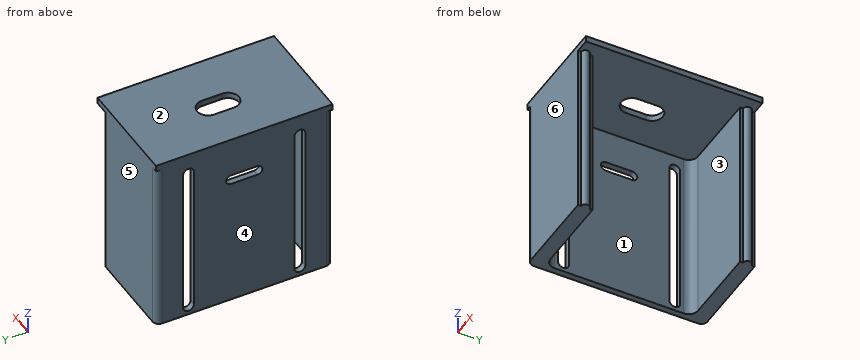
from build123d import *

# Parameters (mm, degrees)
CROQUIS1_W              = 34.637221952
CROQUIS1_H              = 57.24088581
SALIENTE_EXTRUIR1_DEPTH = 2
SALIENTE_EXTRUIR2_DEPTH = 57
CORTAR_EXTRUIR1_DEPTH   = 3
CORTAR_EXTRUIR2_DEPTH   = 6
CORTAR_EXTRUIR3_REACH   = 61


with BuildPart() as part:
    # Croquis1 → Saliente-Extruir1 (new body)
    with BuildSketch(Plane.XY):
        with Locations((-18.894886619, 25.199603339)):
            Rectangle(CROQUIS1_W, CROQUIS1_H)
    extrude(amount=SALIENTE_EXTRUIR1_DEPTH)

    # Croquis3 → Saliente-Extruir2 (add)
    with BuildSketch(Plane(origin=(0, 0, 0), x_dir=(-1, 0, 0), z_dir=(0, 0, -1))):
        with BuildLine():
            Line((6.325110646, 52.869153193), (6.325110646, 53.820046244))
            Line((6.325110646, 53.820046244), (34.213497595, 53.820046244))
            ThreePointArc((34.213497595, 53.820046244), (35.627711158, 53.234259806), (36.213497595, 51.820046244))
            Line((36.213497595, 51.820046244), (36.213497595, -1.420839566))
            ThreePointArc((36.213497595, -1.420839566), (35.627711158, -2.835053128), (34.213497595, -3.420839566))
            Line((34.213497595, -3.420839566), (6.325110646, -3.420839566))
            Line((6.325110646, -3.420839566), (6.325110646, -2.469153193))
            ThreePointArc((6.325110646, -2.469153193), (4.927851766, -1.071894313), (6.325110646, 0.325364567))
            Line((6.325110646, 0.325364567), (6.325110646, 1.27705094))
            Line((6.325110646, 1.27705094), (31.213497595, 1.27705094))
            ThreePointArc((31.213497595, 1.27705094), (33.334817939, 2.155730596), (34.213497595, 4.27705094))
            Line((34.213497595, 4.27705094), (34.213497595, 46.12294906))
            ThreePointArc((34.213497595, 46.12294906), (33.334817939, 48.244269404), (31.213497595, 49.12294906))
            Line((31.213497595, 49.12294906), (6.325110646, 49.12294906))
            Line((6.325110646, 49.12294906), (6.325110646, 50.074635433))
            ThreePointArc((6.325110646, 50.074635433), (4.927851766, 51.471894313), (6.325110646, 52.869153193))
        make_face()
    extrude(amount=SALIENTE_EXTRUIR2_DEPTH)

    # Croquis4 → Cortar-Extruir1 (cut)
    with BuildSketch(Plane.ZY.offset(36.213497595)):
        with BuildLine():
            Line((-5, 41.506708279), (-54, 41.506708279))
            ThreePointArc((-54, 41.506708279), (-55.743291721, 43.25), (-54, 44.993291721))
            Line((-54, 44.993291721), (-5, 44.993291721))
            ThreePointArc((-5, 44.993291721), (-3.256708279, 43.25), (-5, 41.506708279))
        make_face()
        with BuildLine():
            Line((-5, 8.892498399), (-54, 8.892498399))
            ThreePointArc((-54, 8.892498399), (-55.743291721, 7.149206678), (-54, 5.405914957))
            Line((-54, 5.405914957), (-5, 5.405914957))
            ThreePointArc((-5, 5.405914957), (-3.256708279, 7.149206678), (-5, 8.892498399))
        make_face()
    extrude(amount=-CORTAR_EXTRUIR1_DEPTH, mode=Mode.SUBTRACT)

    # Croquis5 → Cortar-Extruir2 (cut)
    with BuildSketch(Plane.ZY.offset(36.213497595)):
        with BuildLine():
            Line((-14.324207984, 20.89), (-14.324207984, 29.51))
            ThreePointArc((-14.324207984, 29.51), (-12.75, 31.084207984), (-11.175792016, 29.51))
            Line((-11.175792016, 29.51), (-11.175792016, 20.89))
            ThreePointArc((-11.175792016, 20.89), (-12.75, 19.315792016), (-14.324207984, 20.89))
        make_face()
    extrude(amount=-CORTAR_EXTRUIR2_DEPTH, mode=Mode.SUBTRACT)

    # Croquis6 → Cortar-Extruir3 (cut, up to next)
    with BuildSketch(Plane.XY.offset(2), mode=Mode.PRIVATE) as cortar_extruir3_sk1:
        with BuildLine():
            Line((-24.042578579, 21.866429816), (-24.042578579, 28.336921124))
            ThreePointArc((-24.042578579, 28.336921124), (-20.515431061, 31.864068642), (-16.988283544, 28.336921124))
            Line((-16.988283544, 28.336921124), (-16.988283544, 21.866429816))
            ThreePointArc((-16.988283544, 21.866429816), (-20.515431061, 18.339282299), (-24.042578579, 21.866429816))
        make_face()
    cortar_extruir3_tool1 = extrude(cortar_extruir3_sk1.sketch, amount=-CORTAR_EXTRUIR3_REACH, mode=Mode.PRIVATE) & part.part
    add(cortar_extruir3_tool1.solids().sort_by_distance((-20.515431, 25.101675, 2))[0], mode=Mode.SUBTRACT)


solid = part.part
Geometry: final body of the model. Coordinates: model frame, mm. Face numbers are marked on the shaded views. A direction names the side the tool comes from. Coordinates: 2 decimals unless noted, no trailing zeros. Order: outer loops, then holes, each group sorted by start corner. A loop starts at its lowest first (then second) coordinate and runs counter-clockwise, first axis right, second up.
1) First-contact query: P1, Ø0.5, axis at y = -3, z = -29, coming from the +X side; P2, Ø5, axis at x = -23, y = 33.5, coming from the -Z side; P3, Ø1, axis at y = 4.5, z = -39.5, coming from the +X side. Flat tips, straight axial feed; report the tip coordinate or a pass-through.
Result sheet:
P1: stops at x = -6.33
P2: stops at z = 0
P3: stops at x = -34.2
2) Section B-B (y = 43.25). Return loops of the section in (x, z).
Result sheet:
outline: (-36.21, -57) - (-34.21, -57) - (-34.21, -55.74) - (-36.21, -55.74) - close; (-36.21, -3.26) - (-34.21, -3.26) - (-34.21, 0) - (-1.58, 0) - (-1.58, 2) - (-36.21, 2) - close
3) Section D-D (y = 25). Return loops of the section in (x, z), then the cut area to 3 significant figures.
Result sheet:
outline: (-36.21, -57) - (-34.21, -57) - (-34.21, -14.32) - (-36.21, -14.32) - close; (-36.21, -11.18) - (-34.21, -11.18) - (-34.21, 0) - (-24.04, 0) - (-24.04, 2) - (-36.21, 2) - close; (-16.99, 0) - (-1.58, 0) - (-1.58, 2) - (-16.99, 2) - close
area: 163 mm2
4) Ray query, probe 1 along Y at (x, z) = (-23.5, -22); probe 2 along X at (y, z) = (17, -38); probe 3 along Z at (x, y) = (-21, 41). Return the intervals inside material, ascending.
Result sheet:
probe 1: y = -3.42 to 1.28, 49.12 to 53.82
probe 2: x = -36.21 to -34.21
probe 3: z = 0 to 2
5) Section C-C (x = -28.5). Return loops of the section in (y, z).
Result sheet:
outline: (-3.42, -57) - (1.28, -57) - (1.28, 0) - (49.12, 0) - (49.12, -57) - (53.82, -57) - (53.82, 2) - (-3.42, 2) - close
6) Set-up query: the marked faces 1 and 2. Return all of +Z, -Z, +X, -X, +Y, -Y with unobstructed straight access to the full face (end or side cutting, diameter ignored); none if empty.
Result sheet:
face 1: -Z, +X
face 2: +Z, +X, -X, +Y, -Y
7) Section A-A (z = -26). Return loops of the section in (x, y), then the cut area to 3 significant figures.
Result sheet:
outline: (-36.21, -1.42) arc R2 ccw to (-34.21, -3.42) - (-6.33, -3.42) - (-6.33, -2.47) arc R1.4 ccw to (-6.33, 0.33) - (-6.33, 1.28) - (-31.21, 1.28) arc R3 cw to (-34.21, 4.28) - (-34.21, 5.41) - (-36.21, 5.41) - close; (-36.21, 8.89) - (-34.21, 8.89) - (-34.21, 41.51) - (-36.21, 41.51) - close; (-36.21, 44.99) - (-34.21, 44.99) - (-34.21, 46.12) arc R3 cw to (-31.21, 49.12) - (-6.33, 49.12) - (-6.33, 50.07) arc R1.4 ccw to (-6.33, 52.87) - (-6.33, 53.82) - (-34.21, 53.82) arc R2 ccw to (-36.21, 51.82) - close
area: 371 mm2
8) Draft query along Y for the marked faces 3, 4, 5 and 6. Return one class per face: released by +Y, released by -Y, zero draft, split by the parting line, or undercut.
Result sheet:
face 3: undercut
face 4: zero draft
face 5: released by +Y
face 6: released by -Y
